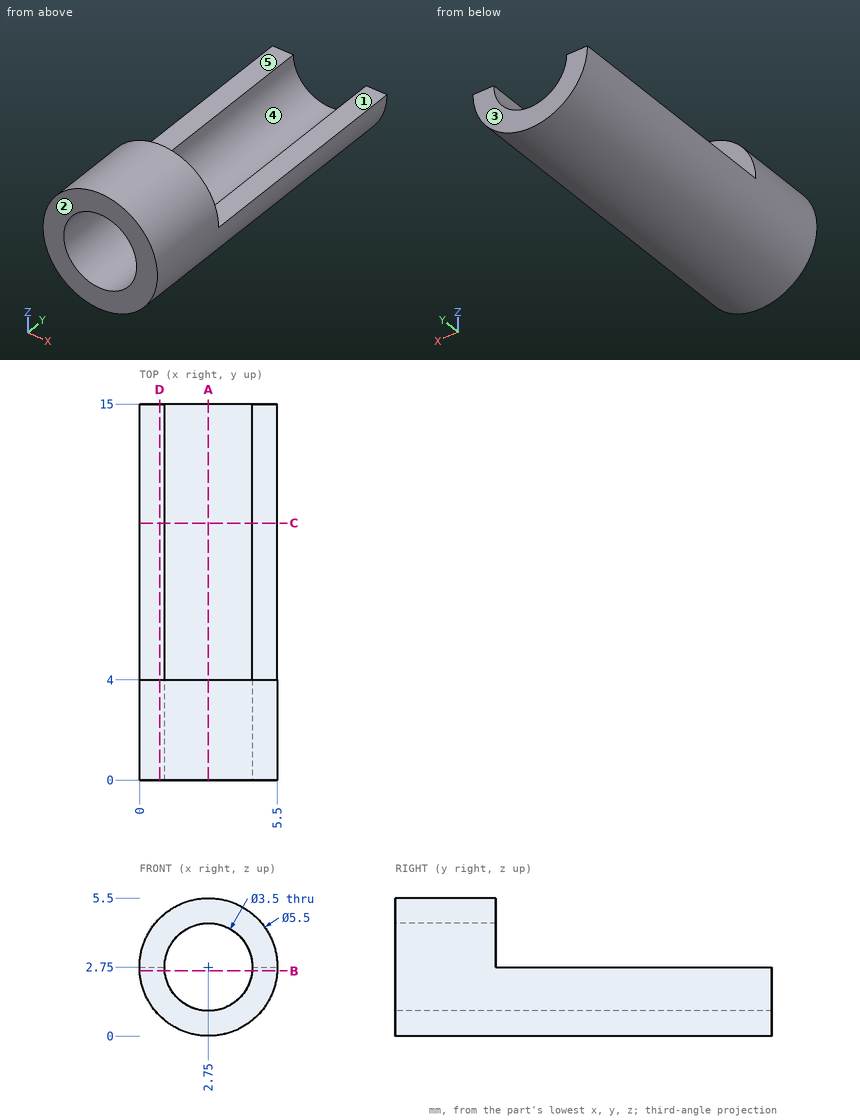
Part print with two shaded views. Sizes in mm from the minimum x, y, z corner. A direction names the side the tool comes from. Round coordinates to 2 decimals unless told otherwise and drop trailing zeros. Order: outer loops, then holes, each group sorted by start corner. A loop starts at its lowest first (then second) coordinate and runs counter-clockwise, first axis right, second up. Notation, with made-up numbers: (54, 43.5) -> (70, 43.5) arc R10 cw to (70, 47.5) -> close; hole circle Ø4 at (70.5, -20). An arc over 180 degrees is marked (long way). Use one line per item in the form item = value.
Item 1: Pull direction Z, two halves, no side cores. Call the marked faces 3, 4 and 5: released by +Z, released by -Z, zero draft, split by the parting line, or undercut.
Returned:
face_3 = zero draft
face_4 = undercut
face_5 = released by +Z
Item 2: Cut at C-C, the plane y = 10.25. Write the cut outline in (x, z), and give its area (3 significant figures).
Returned:
outline = (0, 2.75) arc R2.75 ccw to (5.5, 2.75) -> (4.5, 2.75) arc R1.75 cw to (1, 2.75) -> close
area = 7.07 mm^2
Item 3: Drill centre lines: line 1 (X direction, y = 3.75, z = 2.75); line 2 (Y direction, x = 4.6, z = 3); line 3 (X direction, y = 1.75, z = 1.75). Where is each one in solid material? Low to high.
Returned:
line_1 = 0 to 1, 4.5 to 5.5
line_2 = 0 to 4
line_3 = 0.19 to 1.31, 4.19 to 5.31
Item 4: Tool access for the marked faces 1 and 2: list every direction of +Z, -Z, +X, -X, +Y, -Y with a clear straight run to the whole face (end or side of a thin tool).
Returned:
face_1 = +Z, +X, -X, +Y
face_2 = +Z, -Z, +X, -X, -Y
Item 5: Cut at D-D, the plane x = 0.8. Write the cut outline in (y, z), and give its area (3 significant figures).
Returned:
outline = (0, 0.81) -> (15, 0.81) -> (15, 2.75) -> (4, 2.75) -> (4, 4.69) -> (0, 4.69) -> close
area = 36.8 mm^2
Item 6: Cut at B-B, the plane z = 2.6. Write the cut outline in (x, y), and give its area (3 significant figures).
Returned:
outline = (0, 0) -> (1.01, 0) -> (1.01, 15) -> (0, 15) -> close; (4.49, 0) -> (5.5, 0) -> (5.5, 15) -> (4.49, 15) -> close
area = 30.1 mm^2
Item 7: Flat gauge pins, fed straight in: pin 1 Ø0.8 at (x, z) = (2.5, 4.5) entering from +Y; pin 2 Ø1.5 at (x, y) = (1, 13) entering from +Z. Where does each tip first touch, or does it go through?
Returned:
pin_1 = 4
pin_2 = 2.75
Item 8: Cut at A-A, the plane x = 2.75. Write the cut outline in (y, z), and give its area (3 significant figures).
Returned:
outline = (0, 0) -> (15, 0) -> (15, 1) -> (0, 1) -> close; (0, 4.5) -> (4, 4.5) -> (4, 5.5) -> (0, 5.5) -> close
area = 19.0 mm^2
